Geometry: final body of the model. Coordinates: model frame, mm. Face numbers are marked on the shaded views. A direction names the side the tool comes from. Round coordinates to 2 decimals unless told otherwise and drop trailing zeros. Order: outer loops, then holes, each group sorted by start corner. A loop starts at its lowest first (then second) coordinate and runs counter-clockwise, first axis right, second up. Notation, with made-up numbers: (71, 41.25) - (88, 41.25) arc R12 ccw to (88, 63.25) - close; hole circle Ø6 at (-11.5, -2). An arc over 180 degrees is marked (long way). Put each result on its own line as item: value. Start each with the question number.
(1) Access query for the marked faces 1, 2, 3 and 4. Directions: +Z, -Z, +X, -X, +Y, -Y. A direction counts if a zero-diameter tool reaches every point of the face in a straight line with its end or side. Return the directions, or none.
(2) Pin query (flat end, axial travel): P1, Ø2, axis at x = 62, y = 6, coming from the -Z side; P2, Ø11, axis at x = 89, z = 1, coming from the +Y side; P3, Ø6, axis at y = -2, z = 11.5, coming from the -X side; P4, Ø19, axis at x = 178, z = 0, coming from the -Y side. Return the tip coordinate at first contact, or that it passes through.
(3) Section D-D (x = 0). Output: boundary loops of the cut face in (y, z), and give its area (3 significant figures).
(4) Section A-A (x = 178). Output: boundary loops of the cut face in (y, z), and give its area (3 significant figures).
(5) Section B-B (x = 88). Output: boundary loops of the cut face in (y, z).
(6) Section C-C (y = 16.5). Output: boundary loops of the cut face in (x, z), and give its area (3 significant figures).
(7) Material intervals for L1, parallel to X at y = 2, z = 0; L2, parallel to X at y = 4, z = 0; L3, parallel to X at y = -10.5, z = 0, sorted ascending. Write a range as [from, to].
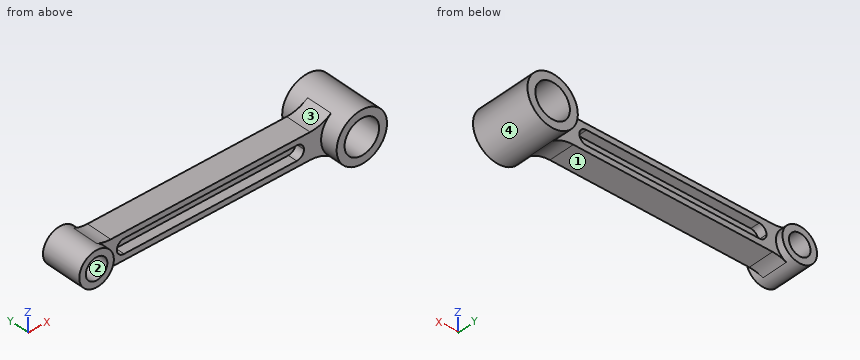
from build123d import *

# Parameters (mm, degrees)
SKETCH1_R           = 17.5
SKETCH1_R_2         = 12
BOSS_EXTRUDE1_DEPTH = 21
SKETCH1_5_R         = 12
SKETCH1_5_R_2       = 7.5
BOSS_EXTRUDE2_DEPTH = 14
BOSS_EXTRUDE3_DEPTH = 9
FILLET2_R           = 24
CUT_EXTRUDE1_START  = -2.5
SKETCH4_W           = 130
SKETCH4_H           = 10
CUT_EXTRUDE1_DEPTH  = 18
FILLET4_R           = 5
FILLET5_R           = 5
FILLET6_R           = 5
FILLET7_R           = 5


with BuildPart() as part:
    # Sketch1 → Boss-Extrude1 (new, symmetric)
    with BuildSketch(Plane(origin=(0, 0, 0), x_dir=(1, 0, 0), z_dir=(0, 1, 0))):
        with Locations(Location((178, 0, 0), (0, 0, 90))):
            Circle(SKETCH1_R)
        with Locations(Location((178, 0, 0), (0, 0, 90))):
            Circle(SKETCH1_R_2, mode=Mode.SUBTRACT)
    extrude(amount=BOSS_EXTRUDE1_DEPTH, both=True)



with BuildPart() as body_2:
    # Sketch1<5> → Boss-Extrude2 (new, symmetric)
    with BuildSketch(Plane(origin=(0, 0, 0), x_dir=(1, 0, 0), z_dir=(0, 1, 0))):
        with Locations(Location((0, 0, 0), (0, 0, 270))):
            Circle(SKETCH1_5_R)
        with Locations(Location((0, 0, 0), (0, 0, 270))):
            Circle(SKETCH1_5_R_2, mode=Mode.SUBTRACT)
    extrude(amount=BOSS_EXTRUDE2_DEPTH, both=True)


with BuildPart() as part_1:
    add(part.part)

    add(body_2.part)  # Boss-Extrude3 merges body 2
    # Sketch2 → Boss-Extrude3 (add, symmetric)
    with BuildSketch(Plane(origin=(0, 0, 0), x_dir=(1, 0, 0), z_dir=(0, 1, 0))):
        with BuildLine():
            Line((7.937253933, 9), (162.99166898, 9))
            ThreePointArc((162.99166898, 9), (160.5, 0), (162.99166898, -9))
            Line((162.99166898, -9), (7.937253933, -9))
            ThreePointArc((7.937253933, -9), (12, 0), (7.937253933, 9))
        make_face()
    extrude(amount=BOSS_EXTRUDE3_DEPTH, both=True)

    # Fillet2
    fillet2_edges = [part_1.edges().sort_by_distance(p)[0] for p in [
        (162.99166898, 0, 9),
        (162.99166898, 0, -9),
        (7.937253933, 0, -9),
        (7.937253933, 0, 9),
    ]]
    fillet(fillet2_edges, radius=FILLET2_R)

    # Sketch4 → Cut-Extrude1 (cut)
    with BuildSketch(Plane(origin=(0, 0, 0), x_dir=(1, 0, 0), z_dir=(0, 1, 0)).offset(CUT_EXTRUDE1_START)):
        with Locations((83.611517753, 0)):
            Rectangle(SKETCH4_W, SKETCH4_H)
    cut_extrude1 = extrude(amount=-CUT_EXTRUDE1_DEPTH, mode=Mode.SUBTRACT)

    # Mirror1: Cut-Extrude1 across plane
    add(cut_extrude1.mirror(Plane.ZX), mode=Mode.SUBTRACT)

    # Fillet4
    fillet4_edges = [part_1.edges().sort_by_distance(p)[0] for p in [
        (18.611517753, 5.75, -5),
        (18.611517753, 5.75, 5),
    ]]
    fillet(fillet4_edges, radius=FILLET4_R - 0.0001)  # a hair under: the kernel refuses the full size

    # Fillet5
    fillet5_edges = [part_1.edges().sort_by_distance(p)[0] for p in [
        (148.611517753, 5.75, 5),
        (148.611517753, 5.75, -5),
    ]]
    fillet(fillet5_edges, radius=FILLET5_R - 0.0001)  # a hair under: the kernel refuses the full size

    # Fillet6
    fillet6_edges = [part_1.edges().sort_by_distance(p)[0] for p in [
        (18.611517753, -5.75, 5),
        (18.611517753, -5.75, -5),
    ]]
    fillet(fillet6_edges, radius=FILLET6_R - 0.0001)  # a hair under: the kernel refuses the full size

    # Fillet7
    fillet7_edges = [part_1.edges().sort_by_distance(p)[0] for p in [
        (148.611517753, -5.75, -5),
        (148.611517753, -5.75, 5),
    ]]
    fillet(fillet7_edges, radius=FILLET7_R - 0.0001)  # a hair under: the kernel refuses the full size


solid = part_1.part
Checks:
1. face 1: -Z, +Y, -Y
1. face 2: +Y, -Y
1. face 3: +Z, +Y, -Y
1. face 4: none
2. P1: stops at z = -9
2. P2: stops at y = 9
2. P3: stops at x = -8.47
2. P4: passes through
3. outline: (-14, -12) - (14, -12) - (14, -7.5) - (-14, -7.5) - close; (-14, 7.5) - (14, 7.5) - (14, 12) - (-14, 12) - close
3. area: 252 mm²
4. outline: (-21, -17.5) - (21, -17.5) - (21, -12) - (-21, -12) - close; (-21, 12) - (21, 12) - (21, 17.5) - (-21, 17.5) - close
4. area: 462 mm²
5. outline: (-9, -9) - (9, -9) - (9, -5) - (2.5, -5) - (2.5, 5) - (9, 5) - (9, 9) - (-9, 9) - (-9, 5) - (-2.5, 5) - (-2.5, -5) - (-9, -5) - close
6. outline: circle Ø35 at (178, 0); hole circle Ø24 at (178, 0)
6. area: 510 mm²
7. L1: x = [-12, -7.5], [7.5, 166], [190, 195.5]
7. L2: x = [-12, -7.5], [7.5, 18.61], [148.61, 166], [190, 195.5]
7. L3: x = [-12, -7.5], [7.5, 12], [160.5, 166], [190, 195.5]
